Geometry: final body of the model. Coordinates: model frame, mm. A direction names the side the tool comes from. Coordinates: 2 decimals unless noted, no trailing zeros. Order: outer loops, then holes, each group sorted by start corner. A loop starts at its lowest first (then second) coordinate and runs counter-clockwise, first axis right, second up. Notation, with made-up numbers: M -4,85.5 L 49,85.5 A26 ccw 49,124.5 Z; hole C 84,81 d4. An arc over 180 degrees is marked long. Use CSV: the item, a comma, the result in double quotes. Start each with the question number.
1. Pull-direction query (X, two-part tool) for faces 1 (the flat face through (10, 0, -15)), 2 (the cylindrical face through (0.46, 0.51, 24.85)), 3 (the cylindrical face through (21.8, 0.5, -18.5)); classes: pulls with the +X half, pulls with the -X half, needs draft (parallel to the pull), parting line crosses it, or undercut.
2. Section query A-A on z = -8.85. Return the cut outline in (x, y) (3 decimals).
3. Set-up query: faces 4 (the flat face through (10, 1, -15)), 5 (the cylindrical face through (-32.59, 0.51, 20.15)). Return all of +Z, -Z, +X, -X, +Y, -Y with unobstructed straight access to the full face (end or side cutting, diameter ignored); none if empty.
4. Section query B-B on x = -24.5. Return the cut outline in (y, z), and give its area (3 significant figures).
5. Section query D-D on z = 24.17. Return the cut outline in (x, y) (3 decimals), and give its area (3 significant figures).
6. Material intervals for line 1 (X direction, y = 0.7, z = -11); line 2 (X direction, y = 0.65, z = -8.85); line 3 (Z direction, x = 16.5, y = 0.85), sorted ascending.
7. Section query C-C on z = 10. Return the cut outline in (x, y), and give its area (3 significant figures).
from build123d import *

# Parameters (mm, degrees)
SKETCH2_W                     = 95
SKETCH2_H                     = 63.5
BOSS_EXTRUDE1_DEPTH           = 1
M3_CLEARANCE_HOLE1_AT_2_COUNT = 2
M3_CLEARANCE_HOLE1_AT_2_PITCH = 48.353205685
M3_CLEARANCE_HOLE1_AT_3_COUNT = 2
M3_CLEARANCE_HOLE1_AT_3_PITCH = 74
M3_CLEARANCE_HOLE1_AT_4_COUNT = 2
M3_CLEARANCE_HOLE1_AT_4_PITCH = 94.757614997
M3_CLEARANCE_HOLE1_AT_5_COUNT = 2
M3_CLEARANCE_HOLE1_AT_5_PITCH = 66.684465957
M3_CLEARANCE_HOLE1_AT_6_COUNT = 2
M3_CLEARANCE_HOLE1_AT_6_PITCH = 52.944922325
CUT_EXTRUDE1_DEPTH            = 1


with BuildPart() as part:
    # Sketch2 → Boss-Extrude1 (new body)
    with BuildSketch(Plane(origin=(0, 0, 0), x_dir=(1, 0, 0), z_dir=(0, 1, 0))):
        Rectangle(SKETCH2_W, SKETCH2_H)
    extrude(amount=BOSS_EXTRUDE1_DEPTH)

    # Sketch8 → M3 Clearance Hole1 (revolve, cut)
    with BuildSketch(Plane(origin=(-39.536732268, 1, -24.17), x_dir=(0, 0, 1), z_dir=(1, 0, 0))):
        Polygon((0, 0), (0, 1), (1.7, 1), (1.7, 0.025), (1.725, 0), align=None)
    m3_clearance_hole1 = revolve(axis=Axis((-39.536732268, 7.35, -24.17), (0, -1, 0)), mode=Mode.SUBTRACT)

    # M3 Clearance Hole1 at 2: M3 Clearance Hole1 ×2
    with Locations(*[Vector(-0.023369701842837577, 0, 0.9997268912236866) * (i * M3_CLEARANCE_HOLE1_AT_2_PITCH) for i in range(1, M3_CLEARANCE_HOLE1_AT_2_COUNT)]):
        add(m3_clearance_hole1, mode=Mode.SUBTRACT)

    # M3 Clearance Hole1 at 3: M3 Clearance Hole1 ×2
    with Locations(*[(i * M3_CLEARANCE_HOLE1_AT_3_PITCH, 0, 0) for i in range(1, M3_CLEARANCE_HOLE1_AT_3_COUNT)]):
        add(m3_clearance_hole1, mode=Mode.SUBTRACT)

    # M3 Clearance Hole1 at 4: M3 Clearance Hole1 ×2
    with Locations(*[Vector(0.8600891865230647, 0, 0.5101436966444779) * (i * M3_CLEARANCE_HOLE1_AT_4_PITCH) for i in range(1, M3_CLEARANCE_HOLE1_AT_4_COUNT)]):
        add(m3_clearance_hole1, mode=Mode.SUBTRACT)

    # M3 Clearance Hole1 at 5: M3 Clearance Hole1 ×2
    with Locations(*[Vector(0.7599970888649028, 0, 0.6499264765470578) * (i * M3_CLEARANCE_HOLE1_AT_5_PITCH) for i in range(1, M3_CLEARANCE_HOLE1_AT_5_COUNT)]):
        add(m3_clearance_hole1, mode=Mode.SUBTRACT)

    # M3 Clearance Hole1 at 6: M3 Clearance Hole1 ×2
    with Locations(*[Vector(0.957221160679124, 0, 0.28935730429368944) * (i * M3_CLEARANCE_HOLE1_AT_6_PITCH) for i in range(1, M3_CLEARANCE_HOLE1_AT_6_COUNT)]):
        add(m3_clearance_hole1, mode=Mode.SUBTRACT)

    # Sketch9 → Cut-Extrude1 (cut)
    with BuildSketch(Plane(origin=(0, 1, 0), x_dir=(1, 0, 0), z_dir=(0, 1, 0))):
        with BuildLine():
            Line((-34.974163292, 19.487383717), (-34.974163292, 22.75))
            ThreePointArc((-34.974163292, 22.75), (-34.095483636, 24.871320344), (-31.974163292, 25.75))
            Line((-31.974163292, 25.75), (-1.684765082, 25.75))
            ThreePointArc((-1.684765082, 25.75), (0.436555262, 24.871320344), (1.315234918, 22.75))
            Line((1.315234918, 22.75), (1.315234918, 7.055031971))
            ThreePointArc((1.315234918, 7.055031971), (2.193914574, 4.933711628), (4.315234918, 4.055031971))
            Line((4.315234918, 4.055031971), (17.971300546, 4.055031971))
            ThreePointArc((17.971300546, 4.055031971), (20.09262089, 4.933711628), (20.971300546, 7.055031971))
            Line((20.971300546, 7.055031971), (20.971300546, 16.428287462))
            ThreePointArc((20.971300546, 16.428287462), (21.849980203, 18.549607805), (23.971300546, 19.428287462))
            Line((23.971300546, 19.428287462), (38.5, 19.428287462))
            ThreePointArc((38.5, 19.428287462), (40.621320344, 18.549607805), (41.5, 16.428287462))
            Line((41.5, 16.428287462), (41.5, -14.560508757))
            ThreePointArc((41.5, -14.560508757), (40.621320344, -16.681829101), (38.5, -17.560508757))
            Line((38.5, -17.560508757), (37.647901029, -17.560508757))
            ThreePointArc((37.647901029, -17.560508757), (35.526580685, -18.439188414), (34.647901029, -20.560508757))
            Line((34.647901029, -20.560508757), (34.647901029, -22.75))
            ThreePointArc((34.647901029, -22.75), (33.769221372, -24.871320344), (31.647901029, -25.75))
            Line((31.647901029, -25.75), (23.971300546, -25.75))
            ThreePointArc((23.971300546, -25.75), (21.849980203, -24.871320344), (20.971300546, -22.75))
            Line((20.971300546, -22.75), (20.971300546, -18.118028913))
            ThreePointArc((20.971300546, -18.118028913), (20.09262089, -15.996708569), (17.971300546, -15.118028913))
            Line((17.971300546, -15.118028913), (4.315234918, -15.118028913))
            ThreePointArc((4.315234918, -15.118028913), (2.193914574, -15.996708569), (1.315234918, -18.118028913))
            Line((1.315234918, -18.118028913), (1.315234918, -22.75))
            ThreePointArc((1.315234918, -22.75), (0.436555262, -24.871320344), (-1.684765082, -25.75))
            Line((-1.684765082, -25.75), (-28.730080623, -25.75))
            ThreePointArc((-28.730080623, -25.75), (-30.851400966, -24.871320344), (-31.730080623, -22.75))
            Line((-31.730080623, -22.75), (-31.730080623, -22.252488185))
            ThreePointArc((-31.730080623, -22.252488185), (-32.608760279, -20.131167841), (-34.730080623, -19.252488185))
            Line((-34.730080623, -19.252488185), (-38.5, -19.252488185))
            ThreePointArc((-38.5, -19.252488185), (-40.621320344, -18.373808528), (-41.5, -16.252488185))
            Line((-41.5, -16.252488185), (-41.5, 13.487383717))
            ThreePointArc((-41.5, 13.487383717), (-40.621320344, 15.60870406), (-38.5, 16.487383717))
            Line((-38.5, 16.487383717), (-37.974163292, 16.487383717))
            ThreePointArc((-37.974163292, 16.487383717), (-35.852842949, 17.366063373), (-34.974163292, 19.487383717))
        make_face()
    extrude(amount=-CUT_EXTRUDE1_DEPTH, mode=Mode.SUBTRACT)


solid = part.part
Results list:
1,face 1,"needs draft"
1,face 2,"undercut"
1,face 3,"undercut"
2,outline,"M -47.5,0 L -41.5,0 L -41.5,1 L -47.5,1 Z; M 1.315,0 L 9.443,0 L 9.443,0.975 L 9.418,1 L 1.315,1 Z; M 12.843,0 L 20.971,0 L 20.971,1 L 12.868,1 L 12.843,0.975 Z; M 41.5,0 L 47.5,0 L 47.5,1 L 41.5,1 Z"
3,face 4,"+Z, -Z, +X, -X, +Y"
3,face 5,"+Y, -Y"
4,outline,"M 0,-31.75 L 1,-31.75 L 1,-25.75 L 0,-25.75 Z; M 0,25.75 L 1,25.75 L 1,31.75 L 0,31.75 Z"
4,area,"12.0 mm²"
5,outline,"M -47.5,0 L -42.367,0 L -42.367,0.975 L -42.392,1 L -47.5,1 Z; M -38.967,0 L -31.373,0 L -31.373,1 L -38.942,1 L -38.967,0.975 Z; M 0.958,0 L 21.329,0 L 21.329,1 L 0.958,1 Z; M 34.291,0 L 40.263,0 L 40.263,0.975 L 40.238,1 L 34.291,1 Z; M 43.663,0 L 47.5,0 L 47.5,1 L 43.688,1 L 43.663,0.975 Z"
5,area,"42.9 mm²"
6,line 1,"x = -47.5 to -41.5, 1.32 to 20.97, 41.5 to 47.5"
6,line 2,"x = -47.5 to -41.5, 1.32 to 9.44, 12.84 to 20.97, 41.5 to 47.5"
6,line 3,"z = -31.75 to -4.06, 15.12 to 31.75"
7,outline,"M -47.5,0 L -41.5,0 L -41.5,1 L -47.5,1 Z; M 41.5,0 L 47.5,0 L 47.5,1 L 41.5,1 Z"
7,area,"12.0 mm²"
